```python
from build123d import *

# Parameters (mm, degrees)
SKETCH1_R           = 4
SKETCH1_R_2         = 1.726448843
SKETCH1_R_3         = 7.5
SKETCH1_R_4         = 1.55
BOSS_EXTRUDE1_DEPTH = 6
SKETCH4_R           = 1.55
CUT_EXTRUDE1_DEPTH  = 3
SKETCH5_R           = 3
CUT_EXTRUDE2_DEPTH  = 59.693125381


with BuildPart() as part:
    # Sketch1 → Boss-Extrude1 (new body)
    with BuildSketch(Plane.XY):
        with BuildLine():
            Line((-44.5, 12.5), (44.5, 12.5))
            ThreePointArc((44.5, 12.5), (57, 0), (44.5, -12.5))
            Line((44.5, -12.5), (-10.829485489, -13.670514511))
            Line((-10.829485489, -13.670514511), (-14.5, -10))
            Line((-14.5, -10), (-52, -10))
            ThreePointArc((-52, -10), (-56.358541226, 3.952847075), (-44.5, 12.5))
        make_face()
        with Locations((10.5, 0)):
            Circle(SKETCH1_R, mode=Mode.SUBTRACT)
        with Locations((15.449747468, 4.949747468)):
            Circle(SKETCH1_R_2, mode=Mode.SUBTRACT)
        with Locations(Location((5.550252532, 4.949747468, 0), (0, 0, 180))):
            Circle(SKETCH1_R_2, mode=Mode.SUBTRACT)
        with Locations((5.550252532, -4.949747468)):
            Circle(SKETCH1_R_2, mode=Mode.SUBTRACT)
        with Locations(Location((15.449747468, -4.949747468, 0), (0, 0, 180))):
            Circle(SKETCH1_R_2, mode=Mode.SUBTRACT)
        with Locations((-19.5, 0)):
            Circle(SKETCH1_R_3, mode=Mode.SUBTRACT)
        with Locations((-5.5, 0)):
            Circle(SKETCH1_R_4, mode=Mode.SUBTRACT)
        with Locations((-33.5, 0)):
            Circle(SKETCH1_R_4, mode=Mode.SUBTRACT)
    extrude(amount=BOSS_EXTRUDE1_DEPTH)

    # Sketch3 → CSK for M5 Flat Head Machine Screw1 (revolve, cut)
    with BuildSketch(Plane(origin=(44.5, 0, 6), x_dir=(0, -1, 0), z_dir=(1, 0, 0))):
        Polygon((0, 0), (0, 6), (2.925, 6), (2.75, 5.825), (2.75, 2.45), (5.2, 0), align=None)
    revolve(axis=Axis((44.5, 0, 12.35), (0, 0, -1)), mode=Mode.SUBTRACT)

    # Sketch4 → Cut-Extrude1 (cut)
    with BuildSketch(Plane.XY.offset(6)):
        with Locations((-43.5, -6)):
            Circle(SKETCH4_R)
        with Locations((-35.5, -6)):
            Circle(SKETCH4_R)
    extrude(amount=-CUT_EXTRUDE1_DEPTH, mode=Mode.SUBTRACT)

    # Sketch5 → Cut-Extrude2 (cut, through all)
    with BuildSketch(Plane.XY.offset(3)):
        with Locations((-35.5, -6)):
            Circle(SKETCH5_R)
        with Locations((-43.5, -6)):
            Circle(SKETCH5_R)
    extrude(amount=-CUT_EXTRUDE2_DEPTH, mode=Mode.SUBTRACT)


solid = part.part
```
Part model, mm, in its own coordinate system. A direction names the side the tool comes from. Coordinates: 2 decimals unless noted, no trailing zeros. Loops run counter-clockwise (first coordinate to the right, second up) from the corner with the lowest first, then second, coordinate; pieces in that order, holes last. Notation, with made-up numbers: (24, 87.5) - (30, 87.5) arc R26 cw to (30, 101.5) - close; hole circle Ø11 at (4, 43.25). An arc over 180 degrees is marked (long way). Write item = value, one per line. Start each with the question number.
Item 1: 3-axis set-ups, long thin cutter, end or side, ignore diameter. For faces 4 (the flat face through (-34, -7, 3)), 5 (the cylindrical face through (-42.022, -5.534, 4.521)), 6 (the flat face through (-33, -10, 3)): which of +Z, -Z, +X, -X, +Y, -Y reach the whole face in a straight line?
Item 2: Cut at A-A, the plane y = 0. Give the cut face in (x, z) (3 decimals), and give its area (3 significant figures).
Item 3: Wall check: L1, parallel to Y at x = -35.5, z = 1.75; L2, parallel to X at y = 0.75, z = 4.9; L3, parallel to Y at x = -43.5, z = 5.05. Give the ranges that are in metal, low to high. Write a range as from..to.
Item 4: Mould opens along Y. For faces 1 (the flat face through (1, 0, 6)), 2 (the cylindrical face through (57, 0, 3)), 3 (the cylindrical face through (-32.022, 0.466, 2.958)) say: released by +Y, released by -Y, zero draft, split by the parting line, or undercut.
Item 5: Cut at B-B, the plane x = 11.5. Give the cut face in (y, z), and give its area (3 significant figures).
Item 6: Cut at D-D, the plane x = -5.5. Give the cut face in (y, z).
Item 7: Flat gauge pins, fed straight in: pin 1 Ø1.5 at (y, z) = (-8.5, 3.5) entering from +X; pin 2 Ø3 at (x, z) = (-31.5, 1.5) entering from -Y; pin 3 Ø3.5 at (x, y) = (-35.5, -6) entering from +Z; pin 4 Ø1 at (y, z) = (4.5, 2.5) entering from +X. Where does each tip first touch, or does it go through?
Item 8: Cut at C-C, the plane z = 1.7. State how many separate pieces and enclosed holes the cut face has, and give its area (3 significant figures).
The answers:
q1.face_4 = -Z
q1.face_5 = +Z, -Z
q1.face_6 = +Z, -Z, -X, -Y
q2.outline = (-57, 0) - (-35.05, 0) - (-35.05, 6) - (-57, 6) - close; (-31.95, 0) - (-27, 0) - (-27, 6) - (-31.95, 6) - close; (-12, 0) - (-7.05, 0) - (-7.05, 6) - (-12, 6) - close; (-3.95, 0) - (6.5, 0) - (6.5, 6) - (-3.95, 6) - close; (14.5, 0) - (41.575, 0) - (41.75, 0.175) - (41.75, 3.55) - (39.3, 6) - (14.5, 6) - close; (47.25, 0.175) - (47.425, 0) - (57, 0) - (57, 6) - (49.7, 6) - (47.25, 3.55) - close
q2.area = 470 mm2
q3.L1 = -10..-9, -3..12.5
q3.L2 = -56.98..-34.86, -32.14..-26.96, -12.04..-6.86, -4.14..6.57, 14.43..40.47, 48.53..56.98
q3.L3 = -10..-7.55, -4.45..12.5
q4.face_1 = zero draft
q4.face_2 = split by the parting line
q4.face_3 = undercut
q5.outline = (-13.2, 0) - (-3.87, 0) - (-3.87, 6) - (-13.2, 6) - close; (3.87, 0) - (12.5, 0) - (12.5, 6) - (3.87, 6) - close
q5.area = 108 mm2
q6.outline = (-13.56, 0) - (-1.55, 0) - (-1.55, 6) - (-13.56, 6) - close; (1.55, 0) - (12.5, 0) - (12.5, 6) - (1.55, 6) - close
q7.pin_1 = 54.31
q7.pin_2 = -10
q7.pin_3 = 6
q7.pin_4 = 56.34
q8.separate_pieces = 1
q8.enclosed_holes = 11
q8.area = 2,300 mm2
